Can you work these out from the model? Positions are in its coordinate system, mm. A direction names the side the tool comes from. Coordinates: 2 decimals unless noted, no trailing zeros. Order: outer loops, then holes, each group sorted by start corner. A loop starts at its lowest first (then second) coordinate and runs counter-clockwise, first axis right, second up. Notation, with made-up numbers: M 37,77 L 79,77 A21 cw 79,98 Z; hole C 88.5,56 d5. An arc over 180 degrees is marked long. Answer as CSV lines item,"result". Start each with the question number.
1. Will these pins go through, and if not, where does the flat tip stop? pin 1 (3 mm diameter, centred on x = 31.02, z = 13.17, fed in from -Y); pin 2 (1 mm diameter, centred on x = -0.5, z = 16, fed in from -Y); pin 3 (6 mm diameter, centred on y = -22, z = 13.17, fed in from +X); pin 4 (4.5 mm diameter, centred on y = -17.5, z = 15, fed in from -X).
2. If we section it at C-C (z = 9.25): List the corners of the cut face in (x, y) for me.
3. If we section it at A-A (y = -5.5): List the corners of the cut face in (x, z) for me.
4. If we section it at B-B (y = -22): List the corners of the cut face in (x, z) for me, plus the area to 3 significant figures.
5. On a 3-axis mill with a long thin cutter (end or side, diameter ignored), from which of +Z, -Z, +X, -X, +Y, -Y can I reach the whole of each face in a straight line? I mean faces 4 (the face through (42.795, -37.817, 13.325)), 5 (the face through (44.03, -25.04, 17.14)). Say none if no direction works.
6. I need wall thicknesses on line 1 along Z through (x, y) = (43.3, -38.5); line 2 along Y through (x, z) = (-9.5, 7.5); line 3 along X through (y, z) = (-24, 15). Which ranges of each line are inside material? Lowest first, please. Write a range as from..to.
7. If we section it at D-D (x = 38): List the corners of the cut face in (y, z) for me, plus the area to 3 significant figures.
8. If we mould it in two halves opening along Y, with no side actions, what happens to faces 1 (the face through (13, 0, 13)), 2 (the face through (43.774, -22, 13)), 3 (the face through (41.274, -23, 13))? For each: released by +Y, released by -Y, zero draft, split by the parting line, or undercut.
```python
from build123d import *

# Parameters (mm, degrees)
SKETCH1_W           = 55
SKETCH1_H           = 15
BOSS_EXTRUDE1_DEPTH = 3
FILLET8_R           = 2
FILLET9_R           = 2
SKETCH2_R           = 1.75
CUT_EXTRUDE1_DEPTH  = 3
SKETCH4_W           = 3
SKETCH4_H           = 15
BOSS_EXTRUDE2_DEPTH = 50
SKETCH6_R           = 0.7
CUT_EXTRUDE2_DEPTH  = 50
SKETCH7_R           = 5
CUT_EXTRUDE3_DEPTH  = 0.5


with BuildPart() as part:
    # Sketch1 → Boss-Extrude1 (new body)
    with BuildSketch(Plane(origin=(0, 0, 0), x_dir=(1, 0, 0), z_dir=(0, 1, 0))):
        with Locations((13.774194124, -13.172794988)):
            Rectangle(SKETCH1_W, SKETCH1_H)
    extrude(amount=BOSS_EXTRUDE1_DEPTH)

    # Fillet8
    fillet8_edges = [part.edges().sort_by_distance(p)[0] for p in [
        (-13.725805876, 1.5, 5.672794988),
    ]]
    fillet(fillet8_edges, radius=FILLET8_R)

    # Fillet9
    fillet9_edges = [part.edges().sort_by_distance(p)[0] for p in [
        (-13.725805876, 1.5, 20.672794988),
    ]]
    fillet(fillet9_edges, radius=FILLET9_R)

    # Sketch2 → Cut-Extrude1 (cut)
    with BuildSketch(Plane(origin=(0, 3, 0), x_dir=(1, 0, 0), z_dir=(0, 1, 0))):
        with Locations((-3.475805876, -13.172794988)):
            Circle(SKETCH2_R)
    cut_extrude1 = extrude(amount=-CUT_EXTRUDE1_DEPTH, mode=Mode.SUBTRACT)

    # Mirror1: Cut-Extrude1 across plane
    add(cut_extrude1.mirror(Plane.ZY.offset(-13.774194124)), mode=Mode.SUBTRACT)

    # Sketch4 → Boss-Extrude2 (add)
    with BuildSketch(Plane(origin=(0, 3, 0), x_dir=(1, 0, 0), z_dir=(0, 1, 0))):
        with Locations((42.774194124, -13.172794988)):
            Rectangle(SKETCH4_W, SKETCH4_H)
    extrude(amount=-BOSS_EXTRUDE2_DEPTH)

    # Sketch6 → Cut-Extrude2 (cut)
    with BuildSketch(Plane(origin=(44.274194124, 0, 0), x_dir=(0, 0, -1), z_dir=(1, 0, 0))):
        with Locations((-13.172794988, -5.5)):
            Circle(SKETCH6_R)
    cut_extrude2 = extrude(amount=-CUT_EXTRUDE2_DEPTH, mode=Mode.SUBTRACT)

    # Mirror2: Cut-Extrude2 across plane
    add(cut_extrude2.mirror(Plane(origin=(0, -22, 0), x_dir=(0, 0, 1), z_dir=(0, -1, 0))), mode=Mode.SUBTRACT)

    # Sketch7 → Cut-Extrude3 (cut)
    with BuildSketch(Plane(origin=(44.274194124, 0, 0), x_dir=(0, 0, -1), z_dir=(1, 0, 0))):
        with Locations((-13.172794988, -22)):
            Circle(SKETCH7_R)
    extrude(amount=-CUT_EXTRUDE3_DEPTH, mode=Mode.SUBTRACT)


solid = part.part
```
Solved:
1,pin 1,"through"
1,pin 2,"y = 0"
1,pin 3,"x = 43.77"
1,pin 4,"x = 41.27"
2,outline,"M -13.73,0 L 41.27,0 L 41.27,-47 L 44.27,-47 L 44.27,-25.1 L 43.77,-25.1 L 43.77,-18.9 L 44.27,-18.9 L 44.27,3 L -13.73,3 Z"
3,outline,"M 41.27,5.67 L 44.27,5.67 L 44.27,12.47 L 41.27,12.47 Z; M 41.27,13.87 L 44.27,13.87 L 44.27,20.67 L 41.27,20.67 Z"
4,outline,"M 41.27,5.67 L 44.27,5.67 L 44.27,8.17 L 43.77,8.17 L 43.77,18.17 L 44.27,18.17 L 44.27,20.67 L 41.27,20.67 Z"
4,area,"40.0 mm²"
5,face 4,"+X, -X"
5,face 5,"+X"
6,line 1,"5.67..12.47, 13.87..20.67"
6,line 2,"0..3"
6,line 3,"41.27..43.77"
7,outline,"M 0,5.67 L 3,5.67 L 3,20.67 L 0,20.67 Z"
7,area,"45.0 mm²"
8,face 1,"released by -Y"
8,face 2,"undercut"
8,face 3,"zero draft"
